The model under review builds one solid part; all positions refer to its coordinate system, in mm. Round coordinates to 2 decimals unless told otherwise and drop trailing zeros. Write each loop counter-clockwise with the first axis right and the second up, starting at its lowest first coordinate (ties: lowest second). Pieces come first, ordered by that corner, then holes. Notation, with made-up numbers: (57, 33.5) - (70, 33.5) arc R17 cw to (70, 47.5) - close; hole circle Ø10 at (36, 74.5). An arc over 180 degrees is marked (long way). One line per question, with ' | ' between items. Start each with the question number.
```python
from build123d import *

# Parameters (mm, degrees)
F1_DEPTH = 50


# Not quite as in the source:
# - a feature names something its author has since deleted; it is built from what else it names


with BuildPart() as f1:
    # F0 (on Front) → F1 (new body)
    with BuildSketch(Plane.XZ):
        with BuildLine():
            Line((0, 0), (0, -120))
            Line((0, -120), (50, -120))
            Line((50, -120), (50, 0.8005096136))
            Line((50, 0.8005096136), (32.5041198008, 0.5203972077))
            Line((32.5041198008, 0.5203972077), (32.7120246633, 10.5182357525))
            ThreePointArc((32.7120246633, 10.5182357525), (25.2401221113, 8.3857971686), (17.7037850617, 10.2779509508))
            Line((17.7037850617, 10.2779509508), (17.4958801992, 0.280112406))
            Line((17.4958801992, 0.280112406), (0, 0))
        make_face()
        with BuildLine():
            ThreePointArc((40, 23.3838750912), (17.3987903619, 36.3152946589), (17.7037850617, 10.2779509508))
            ThreePointArc((17.7037850617, 10.2779509508), (25.2401221113, 8.3857971686), (32.7120246633, 10.5182357525))
            ThreePointArc((32.7120246633, 10.5182357525), (38.0514437889, 15.9906474452), (40, 23.3838750912))
        make_face()
    extrude(amount=F1_DEPTH)


solid = f1.part
```
1. Clearance check with flat-ended pins moving along their axes: P1, Ø4, axis at x = 39.5, y = -39.5, coming from the +Z side; P2, Ø8, axis at x = 7.5, y = -37, coming from the +Z side. State where each tip first meets the part, or that it passes through.
2. The part is to be moulded in two halves that separate along Z. For faces 1 (the face through (25.31, -24.65, 38.38)), 2 (the face through (25, -25, -120)), 3 (the face through (25, -50, -40)), say which applies: pulls with the +Z half, pulls with the -Z half, needs draft (parallel to the pull), parting line crosses it, or undercut.
3. Add section C-C, the plane z = 6. Write out the cut boundary in (x, y).
4. Add section D-D, the plane z = 26. Write out the cut boundary in (x, y).
5. Add section A-A, the plane x = 14.5. Write out the cut boundary in (y, z).
6. Wall thickness on line 1 along Z through (x, y) = (25.5, -18); line 2 along Z through (x, y) = (17, -27); line 3 along Z through (x, y) = (14, -26.5): over which ranges is each line inside the solid? List them lowest first. Write a range as [from, to].
7. Add section B-B, the plane y = -23.5. Write out the cut boundary in (x, z), then the cut area to 3 significant figures.
Geometry check:
1) P1: stops at z = 31.68 | P2: stops at z = 29.92
2) face 1: undercut | face 2: pulls with the -Z half | face 3: needs draft
3) outline: (17.61, -50) - (32.62, -50) - (32.62, 0) - (17.61, 0) - close
4) outline: (10.23, -50) - (39.77, -50) - (39.77, 0) - (10.23, 0) - close
5) outline: (-50, -120) - (0, -120) - (0, 0.23) - (-50, 0.23) - close; (-50, 12.67) - (0, 12.67) - (0, 34.1) - (-50, 34.1) - close
6) line 1: z = [-120, 38.38] | line 2: z = [-120, 0.27], [10.7, 36.07] | line 3: z = [-120, 0.22], [13.19, 33.58]
7) outline: (0, -120) - (50, -120) - (50, 0.8) - (32.5, 0.52) - (32.71, 10.52) arc R15 ccw (long way) to (17.7, 10.28) - (17.5, 0.28) - (0, 0) - close | area: 6,860 mm2
